For this review, take the finished solid that the model builds, in its own axes (mm). Coordinates: 2 decimals unless noted, no trailing zeros. Order: outer loops, then holes, each group sorted by start corner. A loop starts at its lowest first (then second) coordinate and runs counter-clockwise, first axis right, second up. Notation, with made-up numbers: M -24,9.25 L 34,9.25 A30 cw 34,37.25 Z; hole C 67.25,54.5 d4. An arc over 180 degrees is marked long. Use CSV: the item, a comma, the result in double quotes.
```python
from build123d import *

# Parameters (mm, degrees)
SKETCH1_R           = 1.65
BOSS_EXTRUDE1_DEPTH = 5
CUT_EXTRUDE1_DEPTH  = 6


with BuildPart() as part:
    # Sketch1 → Boss-Extrude1 (new body)
    with BuildSketch(Plane.XY):
        with BuildLine():
            Line((-2, -8.31), (2, -8.31))
            ThreePointArc((2, -8.31), (2.707106781, -8.017106781), (3, -7.31))
            Line((3, -7.31), (3, 7.31))
            ThreePointArc((3, 7.31), (2.707106781, 8.017106781), (2, 8.31))
            Line((2, 8.31), (-2, 8.31))
            ThreePointArc((-2, 8.31), (-2.707106781, 8.017106781), (-3, 7.31))
            Line((-3, 7.31), (-3, -7.31))
            ThreePointArc((-3, -7.31), (-2.707106781, -8.017106781), (-2, -8.31))
        make_face()
        with Locations((0, -5.41)):
            Circle(SKETCH1_R, mode=Mode.SUBTRACT)
        with Locations((0, 5.41)):
            Circle(SKETCH1_R, mode=Mode.SUBTRACT)
    extrude(amount=BOSS_EXTRUDE1_DEPTH)

    # Sketch2 → Cut-Extrude1 (cut)
    with BuildSketch(Plane(origin=(3, 0, 0), x_dir=(0, 0, -1), z_dir=(1, 0, 0))):
        with BuildLine():
            Line((-5, -1.3), (-5, 1.3))
            ThreePointArc((-5, 1.3), (-3.7, 0), (-5, -1.3))
        make_face()
    extrude(amount=-CUT_EXTRUDE1_DEPTH, mode=Mode.SUBTRACT)


solid = part.part
```
Item 1: To check wall thickness, follow line 1 along Y through (x, z) = (0, 1.15); line 2 along Y through (x, z) = (0.3, 1.7); line 3 along Y through (x, z) = (-0.35, 4.45). State the ranges of each line that lie inside material, in increasing order. Write a range as [from, to].
Solutions:
line 1,"[-8.31, -7.06], [-3.76, 3.76], [7.06, 8.31]"
line 2,"[-8.31, -7.03], [-3.79, 3.79], [7.03, 8.31]"
line 3,"[-8.31, -7.02], [-3.8, -1.18], [1.18, 3.8], [7.02, 8.31]"
Item 2: Add section A-A on y = 5.41. State the section outline as (x, z) points, and give its area (3 significant figures).
Solutions:
outline,"M -3,0 L -1.65,0 L -1.65,5 L -3,5 Z; M 1.65,0 L 3,0 L 3,5 L 1.65,5 Z"
area,"13.5 mm^2"
Item 3: Add section C-C on z = 2.35. State the section outline as (x, y) points.
Solutions:
outline,"M -3,-7.31 A1 ccw -2,-8.31 L 2,-8.31 A1 ccw 3,-7.31 L 3,7.31 A1 ccw 2,8.31 L -2,8.31 A1 ccw -3,7.31 Z; hole C 0,-5.41 d3.3; hole C 0,5.41 d3.3"
Item 4: Draft analysis for pull direction X (two halves, no side actions). For faces 1 (the face through (-1.31, -6.41, 2.46)), 2 (the face through (3, 0, 2)), 3 (the face through (-1.31, 4.41, 2.46)), 4 (the face through (0, 0, 0)), state which applies: released by +X, released by -X, zero draft, split by the parting line, or undercut.
Solutions:
face 1,"undercut"
face 2,"released by +X"
face 3,"undercut"
face 4,"zero draft"
Item 5: Add section B-B on x = 0. State the section outline as (y, z) points, and give its area (3 significant figures).
Solutions:
outline,"M -8.31,0 L -7.06,0 L -7.06,5 L -8.31,5 Z; M -3.76,0 L 3.76,0 L 3.76,5 L 1.3,5 A1.3 cw -1.3,5 L -3.76,5 Z; M 7.06,0 L 8.31,0 L 8.31,5 L 7.06,5 Z"
area,"47.4 mm^2"
Item 6: Add section D-D on x = -2.6. State the section outline as (y, z) points.
Solutions:
outline,"M -8.11,0 L 8.11,0 L 8.11,5 L 1.3,5 A1.3 cw -1.3,5 L -8.11,5 Z"
Item 7: Clearance check with flat-ended pins moving along their axes: pin 1 Ø1.5 at (x, y) = (2, -6.5) entering from -Z; pin 2 Ø2.5 at (x, y) = (0, 5.41) entering from +Z. State where each tip first meets the part, or that it passes through.
Solutions:
pin 1,"z = 0"
pin 2,"through"
